```python
from build123d import *

# Parameters (mm, degrees)
F1_DEPTH = 300
F2_R     = 3
F3_DEPTH = 50.801
F4_R     = 11
F4_R_2   = 1
F5_DEPTH = 50.801


with BuildPart() as f1:
    # F0 (on Front) → F1 (new body)
    with BuildSketch(Plane.XZ):
        Polygon((0, 50.8), (0, 0), (50.8, 0), (50.8, 1.59), (1.59, 1.59), (1.59, 50.8), align=None)
    extrude(amount=F1_DEPTH)

    # F2 (on Top) → F3 (cut, through all)
    with BuildSketch(Plane.XY):
        with Locations((9.525, -59.525)):
            Circle(F2_R)
        with Locations((9.525, -290.475)):
            Circle(F2_R)
    extrude(amount=F3_DEPTH, mode=Mode.SUBTRACT)

    # F4 (on Right) → F5 (cut, through all)
    with BuildSketch(Plane.YZ):
        with Locations((-25, 25)):
            Circle(F4_R)
        with Locations((-40.5, 9.5)):
            Circle(F4_R_2)
        with Locations((-9.5, 9.5)):
            Circle(F4_R_2)
        with Locations((-9.5, 40.5)):
            Circle(F4_R_2)
        with Locations((-40.5, 40.5)):
            Circle(F4_R_2)
    extrude(amount=F5_DEPTH, mode=Mode.SUBTRACT)


solid = f1.part
```
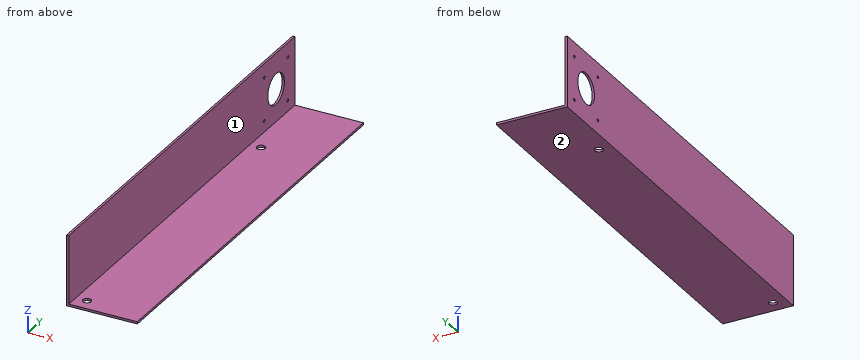
Can you work these out from the model? Positions are in its coordinate system, mm. Face numbers are marked on the shaded views. A direction names the side the tool comes from. Give positions to 0.01 mm unless a question says otherwise; leave off trailing zeros. Write each loop counter-clockwise with the first axis right and the second up, starting at its lowest first coordinate (ties: lowest second). Pieces come first, ordered by that corner, then holes. Notation, with made-up numbers: (14.5, 36.25) - (39.5, 36.25) arc R22 ccw to (39.5, 49.25) - close; hole circle Ø2 at (60.25, 38.5). An arc over 180 degrees is marked (long way). Write item = value, one per line. Start each with the question number.
1. Imagine slicing it at D-D (x = 31.5). Please give me the cut outline in (y, z), and give its area (3 significant figures).
2. Imagine slicing it at A-A (y = -25). Please give me the cut outline in (x, z).
3. Imagine slicing it at C-C (y = -209.5). Please give me the cut outline in (x, z), and give its area (3 significant figures).
4. Please list where these lines run through material, in increasing order: line 1 (Z direction, x = 0.9, y = -9.5); line 2 (Z direction, x = 25, y = -216).
5. Imagine slicing it at B-B (z = 25). Please give me the cut outline in (x, y), and give its area (3 significant figures).
6. On a 3-axis mill with a long thin cutter (end or side, diameter ignored), from which of +Z, -Z, +X, -X, +Y, -Y can I reach the whole of each face in a straight line? I mean the marked faces 1 and 2. Say none if no direction works.
7. For pin 1 (24.5 mm diameter, centred on y = -104.5, z = 29, fed in from +X); pin 2 (15 mm diameter, centred on x = 36, y = -214.5, fed in from +Z), each with a flat end and sliding along its axis, tell me the tip position at first contact or that it passes through.
Worked answers:
q1.outline = (-300, 0) - (0, 0) - (0, 1.59) - (-300, 1.59) - close
q1.area = 477 mm2
q2.outline = (0, 0) - (50.8, 0) - (50.8, 1.59) - (1.59, 1.59) - (1.59, 14) - (0, 14) - close; (0, 36) - (1.59, 36) - (1.59, 50.8) - (0, 50.8) - close
q3.outline = (0, 0) - (50.8, 0) - (50.8, 1.59) - (1.59, 1.59) - (1.59, 50.8) - (0, 50.8) - close
q3.area = 159 mm2
q4.line_1 = 0 to 8.5, 10.5 to 39.5, 41.5 to 50.8
q4.line_2 = 0 to 1.59
q5.outline = (0, -300) - (1.59, -300) - (1.59, -36) - (0, -36) - close; (0, -14) - (1.59, -14) - (1.59, 0) - (0, 0) - close
q5.area = 442 mm2
q6.face_1 = +Z, +X, +Y, -Y
q6.face_2 = -Z, +X, -X, +Y, -Y
q7.pin_1 = 1.59
q7.pin_2 = 1.59
